from build123d import *

# Parameters (mm, degrees)
EXTRUDE_1_DEPTH     = 80
SKETCH_2_R          = 3
CUT_EXTRUDE_1_DEPTH = 85.976467331
SKETCH_3_R          = 3
CUT_EXTRUDE_2_DEPTH = 85.622691992
FILLET_1_R          = 6
FILLET_3_R          = 3


with BuildPart() as part:
    # 草图1 → 凸台-拉伸1 (new body)
    with BuildSketch(Plane.XY):
        Polygon((0, 0), (6, 0), (6, -19), (20, -19), (20, -25), (0, -25), align=None)
    extrude(amount=EXTRUDE_1_DEPTH)

    # 草图2 → 切除-拉伸1 (cut, through all)
    with BuildSketch(Plane(origin=(6, 0, 0), x_dir=(0, 0, -1), z_dir=(1, 0, 0))):
        with Locations(Location((-65, -10, 0), (0, 0, 90))):
            Circle(SKETCH_2_R)
        with Locations(Location((-15, -10, 0), (0, 0, 90))):
            Circle(SKETCH_2_R)
        with Locations(Location((-40, -10, 0), (0, 0, 90))):
            Circle(SKETCH_2_R)
    extrude(amount=-CUT_EXTRUDE_1_DEPTH, mode=Mode.SUBTRACT)

    # 草图3 → 切除-拉伸2 (cut, through all)
    with BuildSketch(Plane(origin=(0, -19, 0), x_dir=(1, 0, 0), z_dir=(0, 1, 0))):
        with Locations(Location((14, -15, 0), (0, 0, 270))):
            Circle(SKETCH_3_R)
        with Locations(Location((14, -65, 0), (0, 0, 270))):
            Circle(SKETCH_3_R)
        with Locations(Location((14, -40, 0), (0, 0, 270))):
            Circle(SKETCH_3_R)
    extrude(amount=-CUT_EXTRUDE_2_DEPTH, mode=Mode.SUBTRACT)

    # 圆角1
    fillet_1_edges = [part.edges().sort_by_distance(p)[0] for p in [
        (0, -25, 40),
    ]]
    fillet(fillet_1_edges, radius=FILLET_1_R)

    # 圆角3
    fillet_3_edges = [part.edges().sort_by_distance(p)[0] for p in [
        (6, -19, 40),
    ]]
    fillet(fillet_3_edges, radius=FILLET_3_R)


solid = part.part
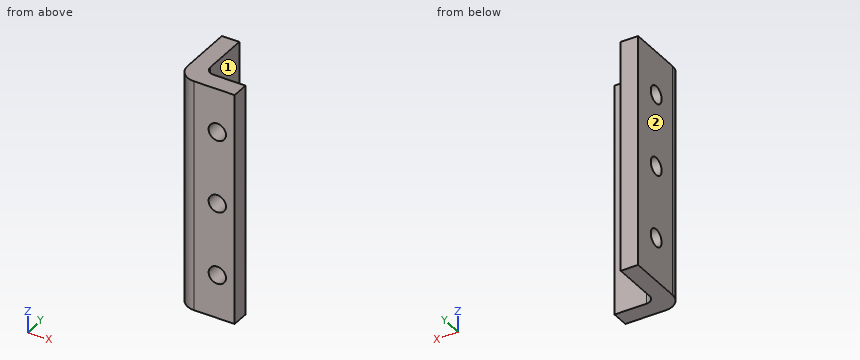
Here's how the part is built. I have some questions about the finished solid (model axes, mm). Face numbers are marked on the shaded views. A direction names the side the tool comes from. Coordinates: 2 decimals unless noted, no trailing zeros. Loops run counter-clockwise (first coordinate to the right, second up) from the corner with the lowest first, then second, coordinate; pieces in that order, holes last.
1. For P1, Ø3.5, axis at x = 14, z = 65, coming from the +Y side; P2, Ø5, axis at x = 15, z = 13, coming from the +Y side; P3, Ø5, axis at y = -5, z = 35.5, coming from the +X side, each with a flat end and sliding along its axis, tell me the tip position at first contact or that it passes through.
2. Imagine slicing it at C-C, the plane y = -10. Please give me the cut outline in (x, z), and give its area (3 significant figures).
3. Imagine slicing it at D-D, the plane z = 52. Please give me the cut outline in (x, y).
4. For the marked faces 1 and 2, which set-ups out of +Z, -Z, +X, -X, +Y, -Y let a thin tool reach every point of the face, with its end or its side?
5. I need wall thicknesses on L1, parallel to Z at x = 4.6, y = -10; L2, parallel to Z at x = 1, y = -9; L3, parallel to X at y = -12, z = 6.5. Which ranges of each line are inside material? Lowest first, please.
6. Imagine slicing it at A-A, the plane x = 14. Please give me the cut outline in (y, z).
7. Imagine slicing it at B-B, the plane z = 15. Please give me the cut outline in (x, y), and give its area (3 significant figures).
Taken from the geometry:
1. P1: passes through
1. P2: stops at y = -19
1. P3: stops at x = 6
2. outline: (0, 0) - (6, 0) - (6, 12) - (0, 12) - close; (0, 18) - (6, 18) - (6, 37) - (0, 37) - close; (0, 43) - (6, 43) - (6, 62) - (0, 62) - close; (0, 68) - (6, 68) - (6, 80) - (0, 80) - close
2. area: 372 mm2
3. outline: (0, -19) arc R6 ccw to (6, -25) - (20, -25) - (20, -19) - (9, -19) arc R3 cw to (6, -16) - (6, 0) - (0, 0) - close
4. face 1: +Z, -Z, +X, +Y
4. face 2: +Z, -Z, -X, +Y, -Y
5. L1: z = 0 to 12, 18 to 37, 43 to 62, 68 to 80
5. L2: z = 0 to 12.17, 17.83 to 37.17, 42.83 to 62.17, 67.83 to 80
5. L3: x = 0 to 6
6. outline: (-25, 0) - (-19, 0) - (-19, 12) - (-25, 12) - close; (-25, 18) - (-19, 18) - (-19, 37) - (-25, 37) - close; (-25, 43) - (-19, 43) - (-19, 62) - (-25, 62) - close; (-25, 68) - (-19, 68) - (-19, 80) - (-25, 80) - close
7. outline: (0, -19) arc R6 ccw to (6, -25) - (11, -25) - (11, -19) - (9, -19) arc R3 cw to (6, -16) - (6, -13) - (0, -13) - close; (0, -7) - (6, -7) - (6, 0) - (0, 0) - close; (17, -25) - (20, -25) - (20, -19) - (17, -19) - close
7. area: 156 mm2
